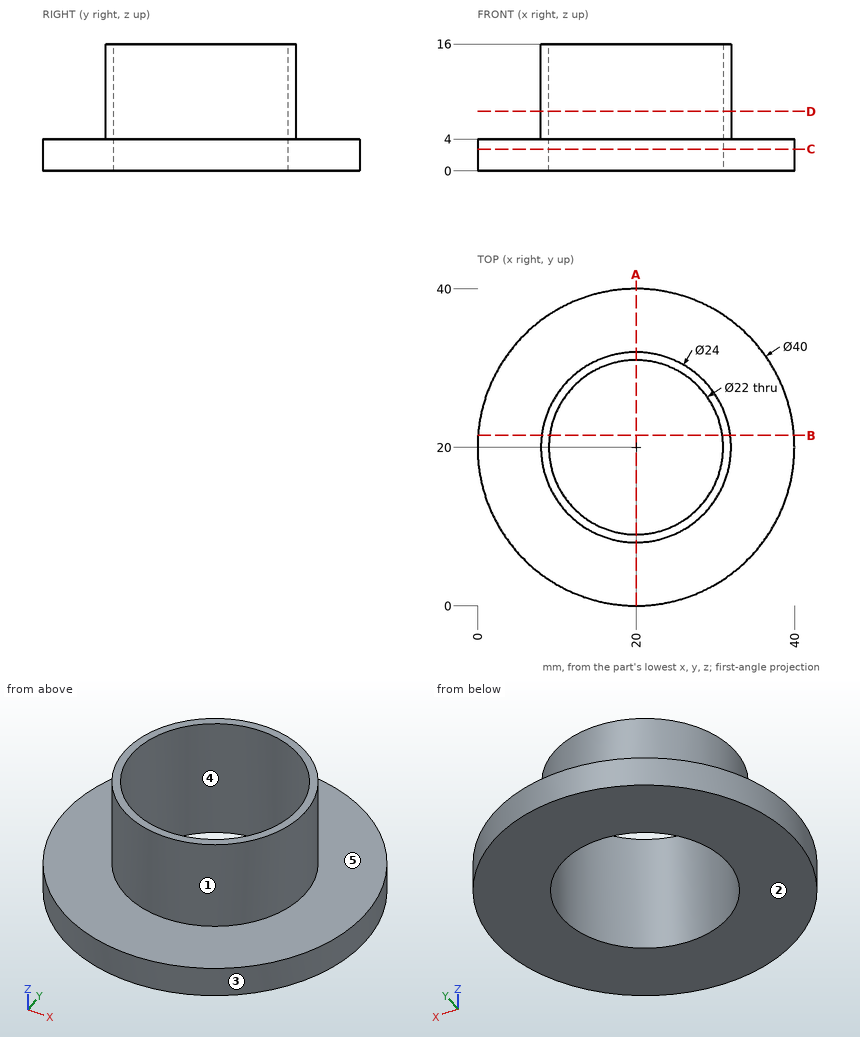
Verification items for this drawing (mm, ordinates from the low corner). A direction names the side the tool comes from. Coordinates: 2 decimals unless noted, no trailing zeros. Write each loop counter-clockwise with the first axis right and the second up, starting at its lowest first coordinate (ties: lowest second). Pieces come first, ordered by that corner, then holes. Notation, with made-up numbers: (65, -7.5) -> (120, -7.5) arc R34 cw to (120, 22.5) -> close; hole circle Ø2 at (-21.75, 13). An arc over 180 degrees is marked (long way). Use CSV: the item, a comma, the result in double quotes. Start each with the question number.
Item 1: Mould release check, pull along Y, two halves, no side actions. Record for the marked faces 3, 4 and 5: released by +Y, released by -Y, zero draft, split by the parting line, or undercut.
Item 2: Cross-section at A-A, the plane x = 20. Record the cut outline in (y, z), plus the area to 3 significant figures.
Item 3: Thickness scan on line 1 (Y direction, x = 20, z = 5.25); line 2 (Y direction, x = 20.5, z = 0.5); line 3 (X direction, y = 19, z = 15.25). Record the ranges inside material, lowest first.
Item 4: Cross-section at C-C, the plane z = 2.75. Record the cut outline in (x, y), plus the area to 3 significant figures.
Item 5: Cross-section at D-D, the plane z = 7.5. Record the cut outline in (x, y), plus the area to 3 significant figures.
Item 6: Depth check by flat-ended pin: pin 1 Ø10 at (x, y) = (18, 10.5) entering from -Z; pin 2 Ø1.5 at (y, z) = (18.5, 3) entering from -X; pin 3 Ø2 at (x, z) = (15.5, 1.5) entering from -Y; pin 4 Ø2 at (y, z) = (10.5, 4.5) entering from +X. Enter the tip coordinate at first touch or a pass-through.
Item 7: Cross-section at B-B, the plane y = 21.5. Record the cut outline in (x, z), plus the area to 3 significant figures.
Item 8: Set-up check for the marked faces 1 and 2: record each of +Z, -Z, +X, -X, +Y, -Y from which the full face is reachable in a straight line by a thin tool's end or side.
Answers:
1,face 3,"split by the parting line"
1,face 4,"undercut"
1,face 5,"zero draft"
2,outline,"(0, 0) -> (9, 0) -> (9, 16) -> (8, 16) -> (8, 4) -> (0, 4) -> close; (31, 0) -> (40, 0) -> (40, 4) -> (32, 4) -> (32, 16) -> (31, 16) -> close"
2,area,"96.0 mm^2"
3,line 1,"8 to 9, 31 to 32"
3,line 2,"0.01 to 9.01, 30.99 to 39.99"
3,line 3,"8.04 to 9.05, 30.95 to 31.96"
4,outline,"circle Ø40 at (20, 20); hole circle Ø22 at (20, 20)"
4,area,"877 mm^2"
5,outline,"circle Ø24 at (20, 20); hole circle Ø22 at (20, 20)"
5,area,"72.3 mm^2"
6,pin 1,"z = 0"
6,pin 2,"x = 0.01"
6,pin 3,"y = 0.31"
6,pin 4,"x = 38.04"
7,outline,"(0.06, 0) -> (9.1, 0) -> (9.1, 16) -> (8.09, 16) -> (8.09, 4) -> (0.06, 4) -> close; (30.9, 0) -> (39.94, 0) -> (39.94, 4) -> (31.91, 4) -> (31.91, 16) -> (30.9, 16) -> close"
7,area,"96.6 mm^2"
8,face 1,"+Z"
8,face 2,"-Z, +X, -X, +Y, -Y"
